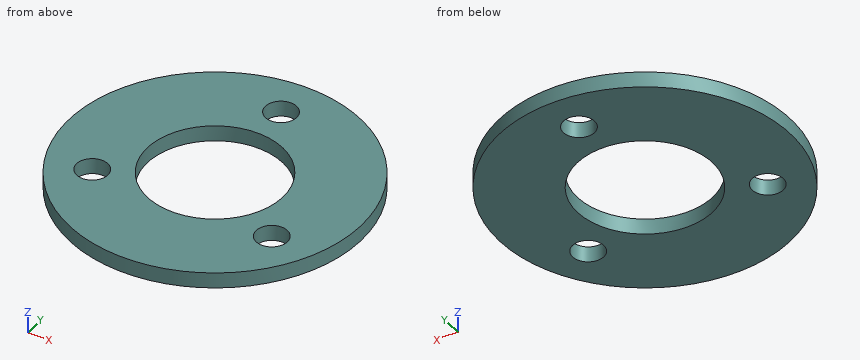
```python
from build123d import *

# Parameters (mm, degrees)
ESBO_O1_R                = 14
ESBO_O1_R_2              = 1.5
ESBO_O1_R_3              = 6.5
RESSALTO_EXTRUS_O1_DEPTH = 1.5


with BuildPart() as part:
    # Esboço1 → Ressalto-extrusão1 (new body)
    with BuildSketch(Plane.XY):
        Circle(ESBO_O1_R)
        with Locations((-8.660254038, -5)):
            Circle(ESBO_O1_R_2, mode=Mode.SUBTRACT)
        with Locations((8.660254038, -5)):
            Circle(ESBO_O1_R_2, mode=Mode.SUBTRACT)
        with Locations((0, 10)):
            Circle(ESBO_O1_R_2, mode=Mode.SUBTRACT)
        Circle(ESBO_O1_R_3, mode=Mode.SUBTRACT)
    extrude(amount=RESSALTO_EXTRUS_O1_DEPTH)


solid = part.part
```
Design review of the part built by this model. Coordinates are the model's own, in mm. Coordinates: 2 decimals unless noted, no trailing zeros. Order: outer loops, then holes, each group sorted by start corner. A loop starts at its lowest first (then second) coordinate and runs counter-clockwise, first axis right, second up.
1) Take a section at A-A, the plane y = 0. Give the boundary of the cut face in (x, z), and give its area (3 significant figures).
2) Take a section at D-D, the plane z = 1.2. Give the boundary of the cut face in (x, y), and give its area (3 significant figures).
3) Wall thickness on line 1 along Y through (x, z) = (0, 1.25); line 2 along X through (y, z) = (-4, 0.65); line 3 along Y through (x, z) = (5, 0.4): over which ranges is each line inside the solid? List them lowest first.
4) Take a section at B-B, the plane x = 0. Give the boundary of the cut face in (y, z).
5) Take a section at C-C, the plane x = 3.75. Give the boundary of the cut face in (y, z), and give its area (3 significant figures).
Returned:
1. outline: (-14, 0) - (-6.5, 0) - (-6.5, 1.5) - (-14, 1.5) - close; (6.5, 0) - (14, 0) - (14, 1.5) - (6.5, 1.5) - close
1. area: 22.5 mm2
2. outline: circle Ø28 at (0, 0); hole circle Ø3 at (-8.66, -5); hole circle Ø13 at (0, 0); hole circle Ø3 at (0, 10); hole circle Ø3 at (8.66, -5)
2. area: 462 mm2
3. line 1: y = -14 to -6.5, 6.5 to 8.5, 11.5 to 14
3. line 2: x = -13.42 to -9.78, -7.54 to -5.12, 5.12 to 7.54, 9.78 to 13.42
3. line 3: y = -13.08 to -4.15, 4.15 to 13.08
4. outline: (-14, 0) - (-6.5, 0) - (-6.5, 1.5) - (-14, 1.5) - close; (6.5, 0) - (8.5, 0) - (8.5, 1.5) - (6.5, 1.5) - close; (11.5, 0) - (14, 0) - (14, 1.5) - (11.5, 1.5) - close
5. outline: (-13.49, 0) - (-5.31, 0) - (-5.31, 1.5) - (-13.49, 1.5) - close; (5.31, 0) - (13.49, 0) - (13.49, 1.5) - (5.31, 1.5) - close
5. area: 24.5 mm2
